Geometry check sheet. Reference: drawing and pictorial views, mm from the part's lowest x, y, z. Round coordinates to 2 decimals unless told otherwise and drop trailing zeros. Order: outer loops, then holes, each group sorted by start corner. A loop starts at its lowest first (then second) coordinate and runs counter-clockwise, first axis right, second up. Notation, with made-up numbers: (-19, 29.5) -> (-6, 29.5) arc R9 cw to (-6, 41.5) -> close; hole circle Ø10 at (38, 24). An arc over 180 degrees is marked (long way). Put each result on its own line as item: value.
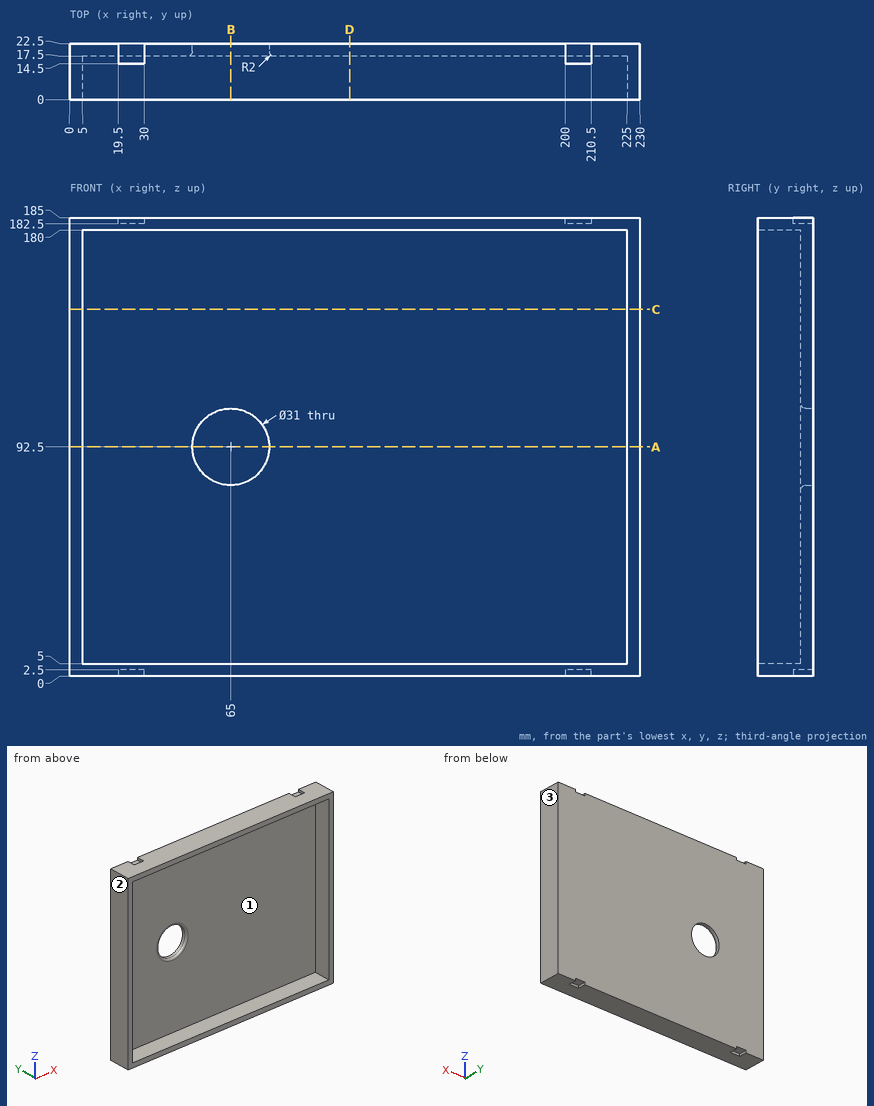
Item 1: Sectioned sample at C-C, the plane z = 148. Record the boundary of the cut face in (x, y), then the cut area to 4 significant figures.
Geometry check:
outline: (0, 0) -> (5, 0) -> (5, 17.5) -> (225, 17.5) -> (225, 0) -> (230, 0) -> (230, 22.5) -> (0, 22.5) -> close
area: 1,325 mm2
Item 2: Sectioned sample at A-A, the plane z = 92.5. Record the boundary of the cut face in (x, y).
Geometry check:
outline: (0, 0) -> (5, 0) -> (5, 17.5) -> (47.5, 17.5) arc R2 ccw to (49.5, 19.5) -> (49.5, 22.5) -> (0, 22.5) -> close; (80.5, 19.5) arc R2 ccw to (82.5, 17.5) -> (225, 17.5) -> (225, 0) -> (230, 0) -> (230, 22.5) -> (80.5, 22.5) -> close
Item 3: Sectioned sample at D-D, the plane x = 113. Record the boundary of the cut face in (y, z), then the cut area to 3 significant figures.
Geometry check:
outline: (0, 0) -> (22.5, 0) -> (22.5, 185) -> (0, 185) -> (0, 180) -> (17.5, 180) -> (17.5, 5) -> (0, 5) -> close
area: 1,100 mm2
Item 4: Release check for a two-part mould opening along X. For the marked faces 1, 2 and 3 record: pulls with the +X half, pulls with the -X half, needs draft (parallel to the pull), parting line crosses it, or undercut.
Geometry check:
face 1: undercut
face 2: pulls with the -X half
face 3: pulls with the +X half
Item 5: Depth check by flat-ended pin: pin 1 Ø12 at (x, y) = (81.5, 10.5) entering from -Z; pin 2 Ø6.5 at (x, y) = (23, 19.5) entering from -Z. Enter the tip coordinate at first touch or a pass-through.
Geometry check:
pin 1: z = 0
pin 2: z = 2.5
Item 6: Material ranges on line 1 along Z through (x, y) = (49.5, 16.75); line 2 along X through (y, z) = (2.25, 15.5); line 3 along Z through (x, y) = (65, 21.8), recorded low to high.
Geometry check:
line 1: 0 to 5, 180 to 185
line 2: 0 to 5, 225 to 230
line 3: 0 to 77, 108 to 185
Item 7: Sectioned sample at B-B, the plane x = 65. Record the boundary of the cut face in (y, z).
Geometry check:
outline: (0, 0) -> (22.5, 0) -> (22.5, 77) -> (19.5, 77) arc R2 ccw to (17.5, 75) -> (17.5, 5) -> (0, 5) -> close; (0, 180) -> (17.5, 180) -> (17.5, 110) arc R2 ccw to (19.5, 108) -> (22.5, 108) -> (22.5, 185) -> (0, 185) -> close
